from build123d import *

# Parameters (mm, degrees)
SKETCH_R          = 25
PAD_DEPTH         = 10
SKETCH001_R       = 28.5
PAD001_DEPTH      = 3
SKETCH002_R       = 4.25
SKETCH002_R_2     = 2.65
POCKET_DEPTH      = 10.501
POCKET_DEPTH_BACK = -2.501
FILLET_R          = 1
FILLET001_R       = 1
CHAMFER_SIZE      = 1


with BuildPart() as part:
    # Sketch → Pad (new body)
    with BuildSketch(Plane.XY):
        Circle(SKETCH_R)
        with BuildLine():
            ThreePointArc((17.347253, -6.023093), (21.799021, 0.111063), (17.133775, 6.08447))
            Line((15, 6.657422), (17.133775, 6.08447))
            Line((15, 14), (15, 6.657422))
            Line((-15, 14), (15, 14))
            Line((-15, 14), (-15, 6.657422))
            Line((-17.133775, 6.08447), (-15, 6.657422))
            ThreePointArc((-17.133775, 6.08447), (-21.799021, 0.111063), (-17.347253, -6.023093))
            Line((-17.347253, -6.023093), (-2.75, -10.5))
            Line((-2.75, -10.5), (2.75, -10.5))
            Line((17.347253, -6.023093), (2.75, -10.5))
        make_face(mode=Mode.SUBTRACT)
    extrude(amount=PAD_DEPTH)

    # Sketch001 (on Face12 of Pad) → Pad001 (join)
    with BuildSketch(Plane(origin=(0, 0, 0), x_dir=(1, 0, 0), z_dir=(0, 0, -1))):
        Circle(SKETCH001_R)
    extrude(amount=PAD001_DEPTH)

    # Sketch002 → Pocket (cut, two sides)
    with BuildSketch(Plane(origin=(0, 0, -0.5), x_dir=(1, 0, 0), z_dir=(0, 0, -1))) as pocket_sk:
        Circle(SKETCH002_R)
        with Locations((-15.75, 0)):
            Circle(SKETCH002_R_2)
        with Locations((15.75, 0)):
            Circle(SKETCH002_R_2)
    extrude(amount=-POCKET_DEPTH, mode=Mode.SUBTRACT)
    extrude(pocket_sk.sketch, amount=-POCKET_DEPTH_BACK, mode=Mode.SUBTRACT)

    # Fillet
    fillet_edges = [part.edges().sort_by_distance(p)[0] for p in [
        (15, 6.657422, 5),
        (15, 14, 5),
        (-15, 6.657422, 5),
        (-15, 14, 5),
        (-2.75, -10.5, 5),
        (2.75, -10.5, 5),
    ]]
    fillet(fillet_edges, radius=FILLET_R)

    # Fillet001
    fillet001_edges = [part.edges().sort_by_distance(p)[0] for p in [
        (0, 14, 10),
        (-15, 10.212165, 10),
        (-21.799021, 0.111063, 10),
        (-10.120283, -8.23957, 10),
        (0, -10.5, 10),
        (10.120283, -8.23957, 10),
        (21.799021, 0.111063, 10),
        (15, 10.212165, 10),
        (14.707107, 13.707107, 10),
        (15.206486, 6.815778, 10),
        (16.437223, 6.271505, 10),
        (-16.437223, 6.271505, 10),
        (-15.206486, 6.815778, 10),
        (-14.707107, 13.707107, 10),
        (-2.748344, -10.488951, 10),
        (2.748344, -10.488951, 10),
    ]]
    fillet(fillet001_edges, radius=FILLET001_R)

    # Chamfer
    chamfer_edges = [part.edges().sort_by_distance(p)[0] for p in [
        (-25, 0, 10),
    ]]
    chamfer(chamfer_edges, length=CHAMFER_SIZE)


solid = part.part
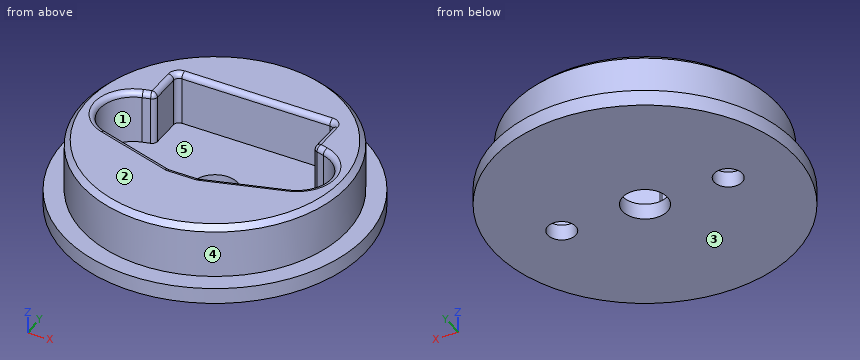
Here's how the part is built. I have some questions about the finished solid (model axes, mm). Face numbers are marked on the shaded views. A direction names the side the tool comes from. Coordinates: 2 decimals unless noted, no trailing zeros. Order: outer loops, then holes, each group sorted by start corner. A loop starts at its lowest first (then second) coordinate and runs counter-clockwise, first axis right, second up. Notation, with made-up numbers: (36, 75) -> (44, 75) arc R12 ccw to (44, 81) -> close; hole circle Ø1 at (-5.5, -1). An arc over 180 degrees is marked (long way). Answer in a Markdown table with one row per item.
(1) I want a section at A-A on x = 0. List the corners of the cut face in (y, z) for me, then the cut area to 3 significant figures.
Answer key:
| item | result |
|---|---|
| outline | (-28.5, -3) -> (-4.25, -3) -> (-4.25, 0) -> (-10.5, 0) -> (-10.5, 9) arc R1 ccw to (-11.5, 10) -> (-24, 10) -> (-25, 9) -> (-25, 0) -> (-28.5, 0) -> close; (4.25, -3) -> (28.5, -3) -> (28.5, 0) -> (25, 0) -> (25, 9) -> (24, 10) -> (15, 10) arc R1 ccw to (14, 9) -> (14, 0) -> (4.25, 0) -> close |
| area | 399 mm^2 |
(2) Will these pins go through, and if not, where does the flat tip stop? pin 1 Ø1 at (x, y) = (-5.5, -9) entering from +Z; pin 2 Ø5 at (x, y) = (0, 0) entering from +Z; pin 3 Ø2.5 at (x, z) = (0, 5) entering from +Y; pin 4 Ø1.5 at (y, z) = (-8, -1.5) entering from -X.
Answer key:
| item | result |
|---|---|
| pin 1 | z = 0 |
| pin 2 | through |
| pin 3 | y = 25 |
| pin 4 | x = -27.56 |
(3) Thinking about a two-plate mould opening in Y: for the marked faces 3, 4 and 5, which applies, +Y half, -Y half, draft (parallel to the pull), parting line (faces both ways), or undercut?
Answer key:
| item | result |
|---|---|
| face 3 | draft |
| face 4 | parting line |
| face 5 | undercut |
(4) I want a section at B-B on z = 5. List the corners of the cut face in (x, y) for me, then the cut area to 3 significant figures.
Answer key:
| item | result |
|---|---|
| outline | circle Ø50 at (0, 0); hole (-17.35, -6.02) -> (-2.89, -10.46) arc R1 ccw to (-2.6, -10.5) -> (2.6, -10.5) arc R1 ccw to (2.89, -10.46) -> (17.35, -6.02) arc R6.3 ccw to (17.13, 6.08) -> (15.74, 6.46) arc R1 cw to (15, 7.42) -> (15, 13) arc R1 ccw to (14, 14) -> (-14, 14) arc R1 ccw to (-15, 13) -> (-15, 7.42) arc R1 cw to (-15.74, 6.46) -> (-17.13, 6.08) arc R6.3 ccw to start |
| area | 1,140 mm^2 |
(5) I want a section at D-D on y = -1. Count the separate pieces of the cut face and the enclosed holes in it, then the cut area to 3 significant figures.
Answer key:
| item | result |
|---|---|
| separate pieces | 4 |
| enclosed holes | 0 |
| area | 180 mm^2 |
(6) I want a section at C-C on z = -1.5. List the corners of the cut face in (x, y) for me.
Answer key:
| item | result |
|---|---|
| outline | circle Ø57 at (0, 0); hole circle Ø5.3 at (-15.75, 0); hole circle Ø8.5 at (0, 0); hole circle Ø5.3 at (15.75, 0) |
(7) On a 3-axis mill with a long thin cutter (end or side, diameter ignored), from which of +Z, -Z, +X, -X, +Y, -Y can I reach the whole of each face in a straight line? I mean the marked faces 1 and 2. Say none if no direction works.
Answer key:
| item | result |
|---|---|
| face 1 | +Z |
| face 2 | +Z, +X, -X, +Y, -Y |
(8) Please list where these lines run through material, in increasing order: probe 1 along X at (y, z) = (0, -2.2); probe 2 along Y at (x, z) = (0, -2.1); probe 3 along X at (y, z) = (2, -1).
Answer key:
| item | result |
|---|---|
| probe 1 | -28.5 to -18.4, -13.1 to -4.25, 4.25 to 13.1, 18.4 to 28.5 |
| probe 2 | -28.5 to -4.25, 4.25 to 28.5 |
| probe 3 | -28.43 to -17.49, -14.01 to -3.75, 3.75 to 14.01, 17.49 to 28.43 |
